Design review of the part built by this model. Coordinates are the model's own, in mm. Face numbers are marked on the shaded views. A direction names the side the tool comes from. Coordinates: 2 decimals unless noted, no trailing zeros. Write each loop counter-clockwise with the first axis right and the second up, starting at its lowest first coordinate (ties: lowest second). Pieces come first, ordered by that corner, then holes.
Q1. Take a section at C-C, the plane x = -14. Write out the cut boundary in (y, z), plus the area to 3 significant figures.
Q2. For L1, parallel to Y at x = -7, z = 8.5; L2, parallel to Y at x = -40, z = -6.65; L3, parallel to Z at x = -19.5, y = 2.5, list the stretches that pass through material, from the lowest coordinate up.
Q3. Take a section at A-A, the plane x = 19.5. Write out the cut boundary in (y, z).
Q4. For the marked faces 4, 5 and 6, list the 3-axis set-ups (+Z, -Z, +X, -X, +Y, -Y) from which the entire face can be reached by the end or side of a thin tool; tool diameter is ignored.
Q5. The part is to be moulded in two halves that separate along Y. For the marked faces 1, 2 and 3, say which applies: released by +Y, released by -Y, zero draft, split by the parting line, or undercut.
Q6. For pin 1 Ø7.5 at (x, y) = (16.5, -3) entering from -Z; pin 2 Ø2.5 at (y, z) = (-2, 0.5) entering from +X; pin 3 Ø1.5 at (y, z) = (-0.5, 6) entering from +X, all flat-tipped, find the tip position at first contact; note any pin that passes through.
Q7. Take a section at B-B, the plane z = -1. Write out the cut boundary in (x, y), plus the area to 3 significant figures.
from build123d import *

# Parameters (mm, degrees)
SKETCH1_W           = 80
SKETCH1_H           = 20
BOSS_EXTRUDE1_DEPTH = 10
SKETCH2_W           = 80
SKETCH2_H           = 7.5
CUT_EXTRUDE1_DEPTH  = 7.5
SKETCH3_R           = 10
BOSS_EXTRUDE2_DEPTH = 10
CHAMFER1_SIZE       = 7.5
SKETCH8_W           = 24.4009661
SKETCH8_H           = 5.102020184
CUT_EXTRUDE2_DEPTH  = 7.5
SKETCH9_R           = 3.8
CUT_EXTRUDE3_DEPTH  = 5
CUT_EXTRUDE4_REACH  = 54.5
SKETCH10_W          = 22
SKETCH10_H          = 13


with BuildPart() as part:
    # Sketch1 → Boss-Extrude1 (new, symmetric)
    with BuildSketch(Plane(origin=(0, 0, 0), x_dir=(1, 0, 0), z_dir=(0, 1, 0))):
        Rectangle(SKETCH1_W, SKETCH1_H)
    extrude(amount=BOSS_EXTRUDE1_DEPTH, both=True)

    # Sketch2 → Cut-Extrude1 (cut, symmetric)
    with BuildSketch(Plane(origin=(0, 0, 0), x_dir=(1, 0, 0), z_dir=(0, 1, 0))):
        with Locations((0, 6.25)):
            Rectangle(SKETCH2_W, SKETCH2_H)
        with Locations((0, -6.25)):
            Rectangle(SKETCH2_W, SKETCH2_H)
    extrude(amount=CUT_EXTRUDE1_DEPTH, both=True, mode=Mode.SUBTRACT)

    # Sketch3 → Boss-Extrude2 (add, symmetric)
    with BuildSketch(Plane.XY):
        with Locations((-40, 0)):
            Circle(SKETCH3_R)
    extrude(amount=BOSS_EXTRUDE2_DEPTH, both=True)

    # Chamfer1
    chamfer1_edges = [part.edges().sort_by_distance(p)[0] for p in [
        (-30, 0, -2.5),
        (-30, 0, 2.5),
    ]]
    chamfer(chamfer1_edges, length=CHAMFER1_SIZE - 0.0001)  # a hair under: the kernel refuses the full size

    # Sketch8 → Cut-Extrude2 (cut)
    with BuildSketch(Plane.XY.offset(10)):
        with Locations((-29.842461096, -0.437762938)):
            Rectangle(SKETCH8_W, SKETCH8_H)
    extrude(amount=-CUT_EXTRUDE2_DEPTH, mode=Mode.SUBTRACT)

    # Sketch9 → Cut-Extrude3 (cut)
    with BuildSketch(Plane(origin=(0, 0, -10), x_dir=(-1, 0, 0), z_dir=(0, 0, -1))):
        with Locations((40, 0)):
            Circle(SKETCH9_R)
    extrude(amount=-CUT_EXTRUDE3_DEPTH, mode=Mode.SUBTRACT)

    # Sketch10 → Cut-Extrude4 (cut, up to next)
    with BuildSketch(Plane(origin=(0, 0, -2.5), x_dir=(-1, 0, 0), z_dir=(0, 0, -1)), mode=Mode.PRIVATE) as cut_extrude4_sk1:
        with Locations((-29, 0)):
            Rectangle(SKETCH10_W, SKETCH10_H)
    cut_extrude4_tool1 = extrude(cut_extrude4_sk1.sketch, amount=-CUT_EXTRUDE4_REACH, mode=Mode.PRIVATE) & part.part
    add(cut_extrude4_tool1.solids().sort_by_distance((29, 0, -2.5))[0], mode=Mode.SUBTRACT)


solid = part.part
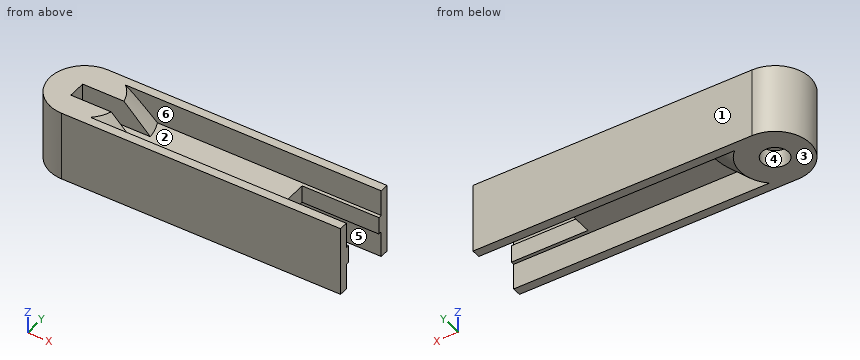
Responses:
1. outline: (-10, -10) - (-7.5, -10) - (-7.5, -2.5) - (7.5, -2.5) - (7.5, -10) - (10, -10) - (10, 10) - (7.5, 10) - (7.5, 2.5) - (-7.5, 2.5) - (-7.5, 10) - (-10, 10) - close
1. area: 175 mm2
2. L1: y = -10 to -7.5, 7.5 to 10
2. L2: y = -10 to -3.8, 3.8 to 10
2. L3: z = -2.5 to 2.5
3. outline: (-10, -10) - (-7.5, -10) - (-7.5, -2.5) - (-6.5, -2.5) - (-6.5, 2.5) - (-7.5, 2.5) - (-7.5, 10) - (-10, 10) - close; (6.5, -2.5) - (7.5, -2.5) - (7.5, -10) - (10, -10) - (10, 10) - (7.5, 10) - (7.5, 2.5) - (6.5, 2.5) - close
4. face 4: -Z
4. face 5: -Z, +X
4. face 6: +Z, +X
5. face 1: released by +Y
5. face 2: undercut
5. face 3: zero draft
6. pin 1: stops at z = -2.5
6. pin 2: stops at x = 18
6. pin 3: stops at x = -42.04
7. outline: (-40, -10) - (40, -10) - (40, -6.5) - (18, -6.5) - (18, 6.5) - (40, 6.5) - (40, 10) - (-40, 10) arc R10 ccw to start
7. area: 1,470 mm2
